```python
from build123d import *

# Parameters (mm, degrees)
F1_DEPTH = 42
F2_W     = 17
F2_H     = 10
F3_DEPTH = 5
F5_DEPTH = 1


with BuildPart() as f1:
    # F0 (on Front) → F1 (new body)
    with BuildSketch(Plane.XZ):
        Polygon((2, 0), (0, 0), (0, 18), (6, 18), (6, 17), (25, 17), (25, 18), (31, 18), (31, 0), (29, 0), (28, -1), (32, -1), (32, 19), (24, 19), (24, 18), (7, 18), (7, 19), (-1, 19), (-1, -1), (3, -1), align=None)
    extrude(amount=F1_DEPTH)

    # F2 (on face) → F3 (cut)
    with BuildSketch(Plane.YZ.offset(32)):
        with Locations((-33.5, 4)):
            Rectangle(F2_W, F2_H)
    extrude(amount=-F3_DEPTH, mode=Mode.SUBTRACT)

    # F4 (on face) → F5 (join)
    with BuildSketch(Plane.XZ.offset(42)):
        Polygon((-1, 9), (32, 9), (32, 19), (24, 19), (24, 18), (7, 18), (7, 19), (-1, 19), align=None)
    extrude(amount=F5_DEPTH)


solid = f1.part
```
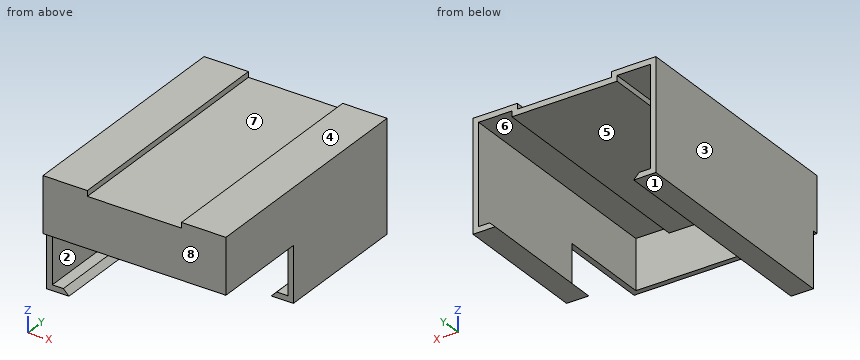
CAD build for the part. Positions are in the model's coordinates, mm. Face numbers are marked on the shaded views. A direction names the side the tool comes from. Round coordinates to 2 decimals unless told otherwise and drop trailing zeros. Order: outer loops, then holes, each group sorted by start corner. A loop starts at its lowest first (then second) coordinate and runs counter-clockwise, first axis right, second up. Notation, with made-up numbers: (-29, 40) - (-16, 40) arc R32 cw to (-16, 69) - close; hole circle Ø2 at (25, 10.25). An arc over 180 degrees is marked (long way). Answer in a Markdown table with one row per item. Add a question column.
(1) Band-saw the part on C-C on x = 11.5. List the corners of the cut face in (y, z), and give its area (3 significant figures).
(2) Probe L1, parallel to X at y = -19.5, z = 12; L2, parallel to Z at x = 16, y = -14; L3, parallel to Y at x = 3.5, z = 16.25. List the from-to ranges inside material, lowest first. Write a range as [from, to].
(3) 3-axis set-ups, long thin cutter, end or side, ignore diameter. For the marked faces 4, 5, 6, 7 and 8: which of +Z, -Z, +X, -X, +Y, -Y reach the whole face in a straight line?
(4) Drop flat-ended pins along their axis: pin 1 Ø5.5 at (x, y) = (18.5, -25) entering from -Z; pin 2 Ø8.5 at (x, y) = (18.5, -29) entering from +Z; pin 3 Ø4 at (x, z) = (27.5, 4) entering from +Y; pin 4 Ø1.5 at (x, z) = (9, 15.5) entering from +Y. Give the stop position or say it passes through.
(5) Mould opens along X. For the marked faces 1, 2 and 3 say: +X half, -X half, draft (parallel to the pull), parting line (faces both ways), or undercut.
(6) Band-saw the part on A-A on z = 4.5. List the corners of the cut face in (x, y), and give its area (3 significant figures).
(7) Band-saw the part on D-D on z = 9.75. List the corners of the cut face in (x, y).
(8) Band-saw the part on B-B on y = -33.5. List the corners of the cut face in (x, z).
Data:
| question | item | result |
|---|---|---|
| 1 | outline | (-43, 9) - (-42, 9) - (-42, 17) - (0, 17) - (0, 18) - (-43, 18) - close |
| 1 | area | 51.0 mm^2 |
| 2 | L1 | x = [-1, 0], [31, 32] |
| 2 | L2 | z = [17, 18] |
| 2 | L3 | y = [-43, -42] |
| 3 | face 4 | +Z, +X, -X, +Y, -Y |
| 3 | face 5 | -Z, +Y |
| 3 | face 6 | +Y |
| 3 | face 7 | +Z, +Y, -Y |
| 3 | face 8 | +Z, -Z, +X, -X, -Y |
| 4 | pin 1 | stops at z = 17 |
| 4 | pin 2 | stops at z = 18 |
| 4 | pin 3 | passes through |
| 4 | pin 4 | stops at y = -42 |
| 5 | face 1 | draft |
| 5 | face 2 | undercut |
| 5 | face 3 | -X half |
| 6 | outline | (-1, -42) - (0, -42) - (0, 0) - (-1, 0) - close; (31, -25) - (32, -25) - (32, 0) - (31, 0) - close |
| 6 | area | 67.0 mm^2 |
| 7 | outline | (-1, -43) - (32, -43) - (32, 0) - (31, 0) - (31, -42) - (0, -42) - (0, 0) - (-1, 0) - close |
| 8 | outline | (-1, -1) - (3, -1) - (2, 0) - (0, 0) - (0, 18) - (6, 18) - (6, 17) - (25, 17) - (25, 18) - (31, 18) - (31, 9) - (32, 9) - (32, 19) - (24, 19) - (24, 18) - (7, 18) - (7, 19) - (-1, 19) - close |
